Input: part model. Units: mm. Frame: model coordinates. Coordinates: 2 decimals unless noted, no trailing zeros. Order: outer loops, then holes, each group sorted by start corner. A loop starts at its lowest first (then second) coordinate and runs counter-clockwise, first axis right, second up.
from build123d import *

# Parameters (mm, degrees)
F0_W     = 177.8
F0_H     = 114.3
F1_DEPTH = 3.175
F2_R     = 7.62
F3_W     = 76.2
F3_H     = 9.525
F4_DEPTH = 25.4
F6_D     = 3.556
F8_D     = 3.81
F11_D    = 3.81
F13_D    = 4.572
F15_D    = 3.81
F16_R    = 57.14999
F18_D    = 3.175


# Not quite as in the source:
# - a fillet or chamfer is up to 0.001 mm smaller than in the source, because OpenCascade refuses the exact size


with BuildPart() as f1:
    # F0 (on Top) → F1 (new body)
    with BuildSketch(Plane.XY):
        with Locations((34.6569041669, 50.5347196277)):
            Rectangle(F0_W, F0_H)
    extrude(amount=F1_DEPTH)

    # F2
    f2_edges = [f1.edges().sort_by_distance(p)[0] for p in [
        (-54.243096, 107.68472, 1.5875),
        (-54.243096, -6.61528, 1.5875),
    ]]
    fillet(f2_edges, radius=F2_R)

    # F3 (on face) → F4 (cut)
    with BuildSketch(Plane.XY.offset(3.175)):
        with Locations((-1.8555958331, -1.8527803723)):
            Rectangle(F3_W, F3_H)
        with Locations((-1.8555958331, 102.9222196277)):
            Rectangle(F3_W, F3_H)
    extrude(amount=-F4_DEPTH, mode=Mode.SUBTRACT)

    # F6 (through all)
    with Locations(Plane.XY.offset(3.175)):
        with Locations((-6.6180958331, 8.8279196277), (-6.6180958331, 46.7755196277), (-6.6180958331, 54.2939196277), (-6.6180958331, 92.2415196277), (6.0819041669, 8.8279196277), (6.0819041669, 46.7755196277), (6.0819041669, 54.2939196277), (6.0819041669, 92.2415196277)):
            Hole(F6_D / 2)

    # F8 (through all)
    with Locations(Plane.XY.offset(3.175)):
        with Locations((32.7773041669, 42.9147196277), (46.2393041669, 42.9147196277), (46.2393041669, 58.1547196277), (32.7773041669, 58.1547196277)):
            Hole(F8_D / 2)

    # F11 (through all)
    with Locations(Plane.XY.offset(3.175)):
        with Locations((-22.4930958331, 31.4847196277), (-22.4930958331, 69.5847196277)):
            Hole(F11_D / 2)

    # F13 (through all)
    with Locations(Plane.XY.offset(3.175)):
        with Locations((76.4399041669, 65.6477196277), (76.4399041669, 35.4217196277), (100.8239041669, 35.4217196277), (100.8239041669, 65.6477196277)):
            Hole(F13_D / 2)

    # F15 (through all)
    with Locations(Plane.XY.offset(3.175)):
        with Locations((-19.3180958331, 12.4347196277), (-19.3180958331, 88.6347196277), (56.8819041669, 88.6347196277), (56.8819041669, 12.4347196277)):
            Hole(F15_D / 2)

    # F16 (radius 57.15 in the source; OpenCascade refuses exactly that, so slightly less here)
    f16_edges = [f1.edges().sort_by_distance(p)[0] for p in [
        (123.556904, -6.61528, 1.5875),
        (123.556904, 107.68472, 1.5875),
    ]]
    fillet(f16_edges, radius=F16_R)

    # F18 (through all)
    with Locations(Plane.XY.offset(3.175)):
        with Locations((81.0781642795, 2.9097196277), (90.9841642795, 25.0077196277), (90.9841642795, 76.0617196277), (81.0781642795, 98.1597196277)):
            Hole(F18_D / 2)


solid = f1.part
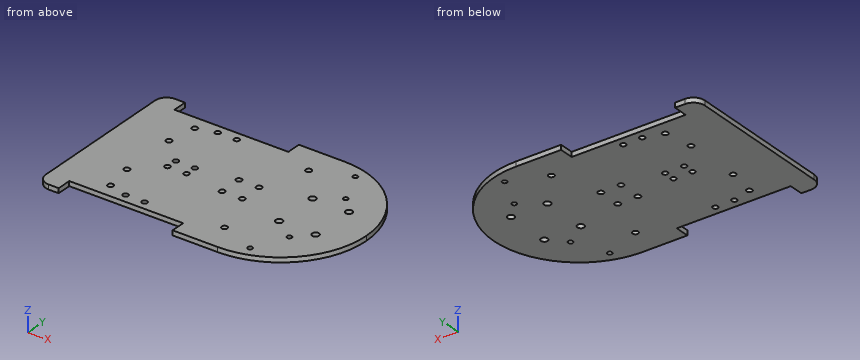
Item 1: Cut plane C-C on z = 2.4. Count the separate pieces of the cut face and the enclosed holes in it, then the cut area to 3 significant figures.
Response values:
separate pieces: 1
enclosed holes: 26
area: 17,200 mm2
Item 2: Ray query, probe 1 along Y at (x, z) = (80, 1.45); probe 2 along Y at (x, z) = (-24, 2.05); probe 3 along X at (y, z) = (44.5, 1.3). Return the intervals inside material, ascending.
Response values:
probe 1: y = -4.98 to 1.74, 4.07 to 96.99, 99.32 to 106.04
probe 2: y = 2.91 to 30.32, 32.65 to 68.42, 70.75 to 98.16
probe 3: x = -54.24 to 31.72, 33.83 to 45.18, 47.3 to 123.24
Item 3: Cut plane A-A on y = 84.5. Return loops of the section in (x, z) (3 decimals).
Response values:
outline: (-54.243, 0) - (112.369, 0) - (112.369, 3.175) - (-54.243, 3.175) - close
Item 4: Pin query (flat end, axial travel): pin 1 Ø2.5 at (x, y) = (-22.49, 69.58) entering from +Z; pin 2 Ø1.5 at (y, z) = (45, 2) entering from +X; pin 3 Ø1 at (x, z) = (-7.5, 1.5) entering from +Y; pin 4 Ø1.5 at (x, z) = (97.5, 0.5) entering from +Y. Return the tip coordinate at first contact, or that it passes through.
Response values:
pin 1: passes through
pin 2: stops at x = 123.36
pin 3: stops at y = 98.16
pin 4: stops at y = 98.96
Item 5: Cut plane B-B on x = 2.5. Return loops of the section in (y, z) (3 decimals), then the cut area to 3 significant figures.
Response values:
outline: (2.91, 0) - (98.16, 0) - (98.16, 3.175) - (2.91, 3.175) - close
area: 302 mm2
